Source: CAD feature listing. Evaluate the final solid. Frame: model axes, mm. Face numbers are marked on the shaded views. A direction names the side the tool comes from. Round coordinates to 2 decimals unless told otherwise and drop trailing zeros. Write each loop counter-clockwise with the first axis right and the second up, starting at its lowest first coordinate (ties: lowest second). Pieces come first, ordered by that corner, then holes. Notation, with made-up numbers: M 7,62 L 36,62 A16 cw 36,89 Z; hole C 31,-33.5 d9. An arc over 180 degrees is marked long. Use a Markdown table: item, result.
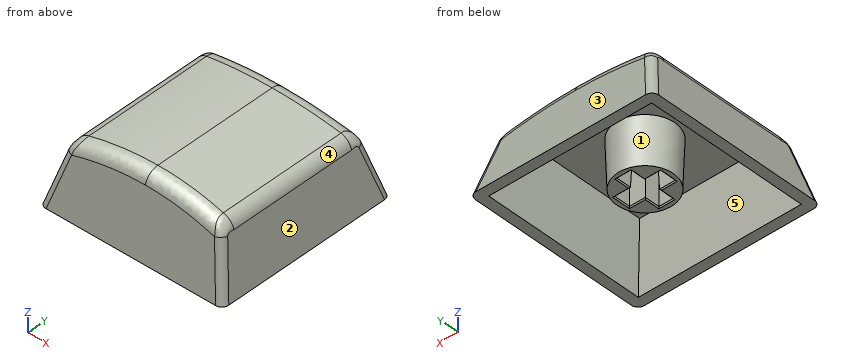
Autodesk Fusion 360 part; units mm, degrees
sketch "Stem dimensions" plane through (0, 0, 0) normal (0, 0, 1) x (1, 0, 0)
  line L0 (0, 0) -> (4, 0)
  line L1 (4, 0) -> (4, 1.3)
  line L2 (4, 1.3) -> (0, 1.3)
  line L3 (0, 1.3) -> (0, 0)
  line L4 (1.45, 2.65) -> (2.55, 2.65)
  line L5 (2.55, 2.65) -> (2.55, -1.35)
  line L6 (2.55, -1.35) -> (1.45, -1.35)
  line L7 (1.45, -1.35) -> (1.45, 2.65)
  line L8 (0, 1.3) -> (4, 0) construction
  line L9 (0, 0) -> (4, 1.3) construction
  line L10 (2, -1.35) -> (2, 2.65) construction
  line L11 (2.55, 0.65) -> (1.45, 0.65) construction
  point P0 (2, 0.65)
  point P1 (2, 0.65)
  point P2 (2, 0.65)
  dimension "d1" = 4
  dimension "d2" = 1.3
  dimension "d3" = 1.1
  dimension "d4" = 4
sketch "Stem clearance" plane through (0, 0, 0) normal (0, 0, 1) x (1, 0, 0)
  line L0 (4, 1.3) -> (0, 1.3) construction
  line L1 (1.45, -1.35) -> (1.45, 2.65) construction
  line L2 (1.45, 2.65) -> (2.55, 2.65) construction
  line L3 (2.55, 2.65) -> (2.55, -1.35) construction
  line L4 (4, 0) -> (4, 1.3) construction
  line L5 (0, 0) -> (4, 0) construction
  line L6 (2.55, -1.35) -> (1.45, -1.35) construction
  line L7 (0, 1.3) -> (0, 0) construction
  line L8 (-0.25, 1.45) -> (1.3, 1.45)
  line L9 (1.3, 1.45) -> (1.3, 2.9)
  line L10 (1.3, 2.9) -> (2.7, 2.9)
  line L11 (2.7, 2.9) -> (2.7, 1.45)
  line L12 (2.7, 1.45) -> (4.25, 1.45)
  line L13 (4.25, 1.45) -> (4.25, -0.15)
  line L14 (4.25, -0.15) -> (2.7, -0.15)
  line L15 (2.7, -0.15) -> (2.7, -1.6)
  line L16 (2.7, -1.6) -> (1.3, -1.6)
  line L17 (1.3, -1.6) -> (1.3, -0.15)
  line L18 (1.3, -0.15) -> (-0.25, -0.15)
  line L19 (-0.25, -0.15) -> (-0.25, 1.45)
  circle A0 centre (2, 0.65) radius 2.75
  point P0 (2, 0.65)
  dimension "gap" = 0.15
  dimension "gap_edge" = 0.25
  dimension "d7" = 0.15
  dimension "d8" = 0.25
  dimension "d9" = 0.25
  dimension "d10" = 0.25
  dimension "d11" = 0.15
  dimension "d12" = 0.15
  dimension "d13" = 5.5
ref_plane "WorkPlane1" through (2, 0.65, 0) normal (1, 0, 0) x (0, 1, 0)
sketch "Stem - vertical" plane through (2, 0, 0) normal (1, 0, 0) x (0, 1, 0)
  line L0 (-1.35, 0) -> (2.65, 0) construction
  line L1 (0.65, 0) -> (0.65, 5.6)
  point P0 (0.65, 1)
  point P1 (0.65, 0)
  dimension "d16" = 1
  dimension "d28" = 4.6
extrude "Extrude1" add sketch "Stem clearance" along normal up to surface (4.6 mm away) draft 2 from surface at 1 makes body 1
chamfer "Chamfer1" distance 0.1 angle 45 12 edges at (1.3, -0.875, 1) (2, -1.6, 1) (2.7, -0.875, 1) (3.475, -0.15, 1) (4.25, 0.65, 1) (3.475, 1.45, 1) (2.7, 2.175, 1) (2, 2.9, 1) (1.3, 2.175, 1) (0.525, 1.45, 1) (-0.25, 0.65, 1) (0.525, -0.15, 1) on bodies 1
sketch "Keycap bottom" plane through (0, 0, 0) normal (0, 0, 1) x (1, 0, 0)
  line L0 (2.55, 0.65) -> (1.45, 0.65) construction
  line L1 (2, -1.35) -> (2, 2.65) construction
  line L2 (-7, -8.35) -> (11, -8.35)
  line L3 (11, -8.35) -> (11, 9.65)
  line L4 (11, 9.65) -> (-7, 9.65)
  line L5 (-7, 9.65) -> (-7, -8.35)
  line L6 (-7, 9.65) -> (11, -8.35) construction
  line L7 (11, 9.65) -> (-7, -8.35) construction
  line L8 (-6, -7.35) -> (10, -7.35)
  line L9 (10, -7.35) -> (10, 8.65)
  line L10 (10, 8.65) -> (-6, 8.65)
  line L11 (-6, 8.65) -> (-6, -7.35)
  point P0 (2, 0.65)
  point P1 (2, 0.65)
  dimension "keycap_size" = 18
  dimension "d21" = 18
  dimension "d29" = 16
ref_plane "WorkPlane2" through (2, 0.65, 0) normal (0, 1, 0) x (-1, 0, 0)
extrude "Extrude2" add sketch "Keycap bottom" along normal blind 12 separate body contours L2 L3 L4 L5 | L8 L9 L10 L11 makes body 2
sketch "Keycap front-back profile" plane through (0, 0.65, 0) normal (0, 1, 0) x (1, 0, 0)
  line L0 (4.9106, -5.6) -> (-0.9106, -5.6) construction
  line L1 (-7, 0) -> (11, 0)
  line L2 (2, -5.6) -> (2, 23.2) construction
  arc A0 (-17.02, 0) -> (2, -6.8) centre (2, 23.2) ccw
  line L3 (-7, 0) -> (-5.4283, -5.8658)
  arc A1 (2, -6.8) -> (21.02, 0) centre (2, 23.2) ccw
  line L4 (11, 0) -> (9.4283, -5.8658)
  point P0 (-6, 0)
  point P1 (10, 0)
  dimension "d31" = 1.2
  dimension "d32" = 75
  dimension "d46" = 30
extrude "Extrude4" cut sketch "Keycap front-back profile" along normal through all and the other way through all keep common part bodies 2 1
sketch "Keycap left-right profile" plane through (2, 0, 0) normal (1, 0, 0) x (0, 1, 0)
  line L0 (-8.35, 0) -> (9.65, 0)
  line L1 (-2.2606, 5.6) -> (3.5606, 5.6) construction
  line L2 (-8.35, 0) -> (-6.5279, 6.8)
  line L3 (-6.5279, 6.8) -> (0.65, 6.8)
  line L4 (0.65, 5.6) -> (0.65, -23.2)
  line L5 (7.8279, 6.8) -> (0.65, 6.8)
  line L6 (9.65, 0) -> (7.8279, 6.8)
  point P0 (8.65, 0)
  point P1 (-7.35, 0)
  point P2 (0.65, 6.8)
  dimension "d40" = 75
extrude "Extrude5" cut sketch "Keycap left-right profile" along normal through all and the other way through all keep common part bodies 2 1
fillet "Fillet1" radius 1.4 4 edges at (9.4283, 0.65, 5.8658) (-5.4283, 0.65, 5.8658) (2, 7.8279, 6.8) (2, -6.5279, 6.8) on bodies 2
fillet "Fillet1" radius 0.7 4 edges at (10.2141, 8.8641, 2.9329) (-6.2141, 8.8641, 2.9329) (-6.2141, -7.5641, 2.9329) (10.2141, -7.5641, 2.9329) on bodies 2
extrude "Extrude3" cut sketch "Keycap bottom" along normal up to surface (5.6 mm away) draft -15 contours L8 L9 L10 L11 bodies 2
combine "Combine1" operation add target body 2 tool bodies 1
equation "d7 = gap"
equation "d8 = gap_edge"
equation "d9 = gap_edge"
equation "d10 = gap_edge"
equation "d11 = gap"
equation "d12 = gap"
equation "d21 = keycap_size"
equation "d28 = 4 mm + 0.6 mm"
equation "d40 = d32"
Q1. Section C-C on y = -5. Return loops of the section in (x, z), plus the area to 3 significant figures.
Results are:
| item | result |
|---|---|
| outline | M -7,0 L -6,0 L -4.5,5.6 L 8.5,5.6 L 10,0 L 11,0 L 9.64,5.06 A1.4 ccw 8.6,6.07 A30 ccw 2,6.8 A30 ccw -4.6,6.07 A1.4 ccw -5.64,5.06 Z |
| area | 24.2 mm^2 |
Q2. Mould query, pull axis Y, two halves, no side actions, for the marked faces 1, 2 and 3. Classes: +Y half, -Y half, draft (parallel to the pull), parting line (faces both ways), or undercut.
Results are:
| item | result |
|---|---|
| face 1 | undercut |
| face 2 | draft |
| face 3 | +Y half |
Q3. First-contact query: pin 1 Ø2 at (x, y) = (5, 4) entering from -Z; pin 2 Ø8 at (x, y) = (5.5, 0) entering from -Z; pin 3 Ø1 at (y, z) = (-4.5, 1) entering from +X; pin 4 Ø3 at (x, z) = (-5, 1) entering from -Y. Flat tips, straight axial feed; report the tip coordinate or a pass-through.
Results are:
| item | result |
|---|---|
| pin 1 | z = 5.6 |
| pin 2 | z = 1 |
| pin 3 | x = 10.87 |
| pin 4 | y = -8.35 |
Q4. Section A-A on y = 0.65. Return loops of the section in (x, z).
Results are:
| item | result |
|---|---|
| outline | M -7,0 L -6,0 L -4.5,5.6 L -0.91,5.6 L -0.75,1 L -0.35,1 L -0.25,1.1 L -0.09,5.6 L 4.09,5.6 L 4.25,1.1 L 4.35,1 L 4.75,1 L 4.91,5.6 L 8.5,5.6 L 10,0 L 11,0 L 9.64,5.06 A1.4 ccw 8.6,6.07 A30 ccw 2,6.8 A30 ccw -4.6,6.07 A1.4 ccw -5.64,5.06 Z |
Q5. Reachability of the marked faces 4 and 5 from +Z, -Z, +X, -X, +Y, -Y: full face, straight path, thin tool, end or side. Return the list, or none.
Results are:
| item | result |
|---|---|
| face 4 | +Z, +X, +Y, -Y |
| face 5 | -Z |
Q6. Line query: L1, parallel to X at y = 3.25, z = 5.5; L2, parallel to X at y = 0, z = 2.75; L3, parallel to Y at x = 2.25, z = 2. Output: solid intervals per line, ascending.
Results are:
| item | result |
|---|---|
| L1 | -5.44 to -4.53, 0.7 to 3.3, 8.53 to 9.44 |
| L2 | -6.26 to -5.26, -0.73 to -0.19, 4.19 to 4.73, 9.26 to 10.26 |
| L3 | -7.81 to -6.81, -2.12 to -1.57, 2.87 to 3.42, 8.11 to 9.11 |
Q7. Section B-B on z = 3.75. Give the number of separate pieces and of enclosed holes in the cut face, plus the area to 3 significant figures.
Results are:
| item | result |
|---|---|
| separate pieces | 2 |
| enclosed holes | 2 |
| area | 75.5 mm^2 |
